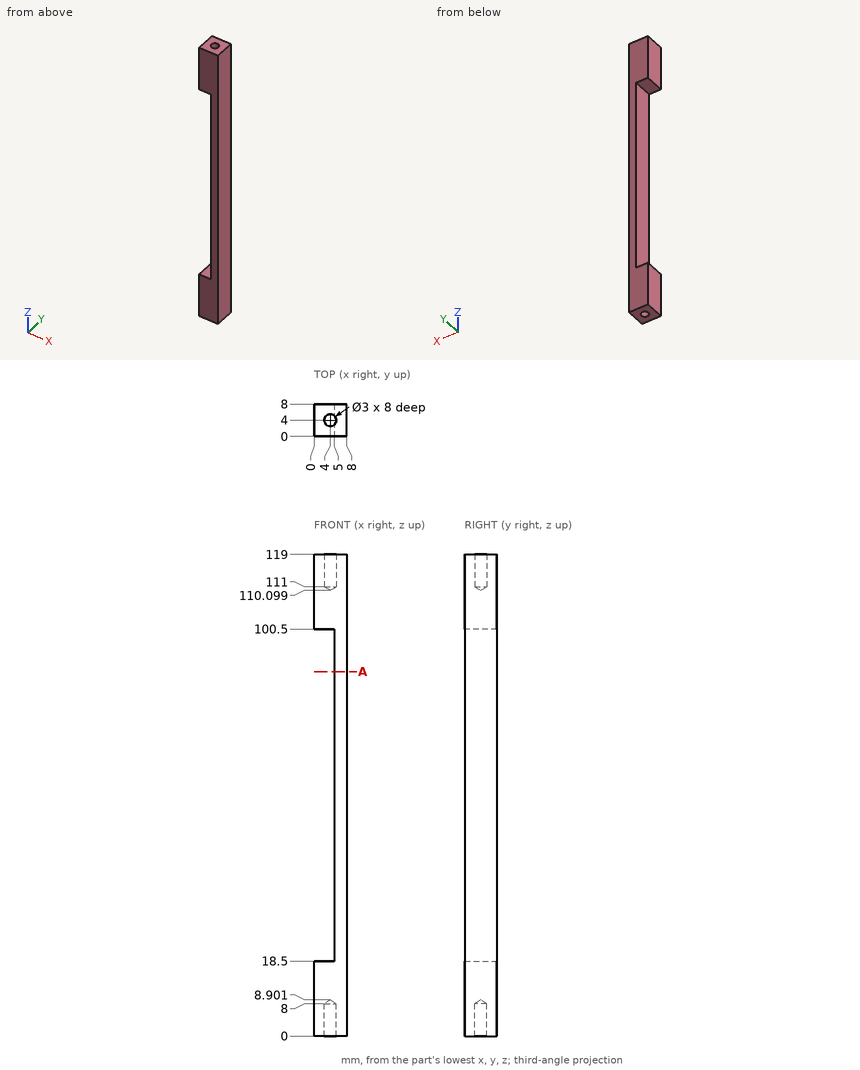
Can you work these out from the drawing? Everything is in mm from the part's minimum corner. Give positions to 0.01 mm unless a question says otherwise; leave off trailing zeros. Loops run counter-clockwise (first coordinate to the right, second up) from the corner with the lowest first, then second, coordinate; pieces in that order, holes last. Notation, with made-up numbers: M 62,54 L 109,54 A12 cw 109,71 Z; hole C 14.5,72.5 d1. An arc over 180 degrees is marked long. Put each result on its own line as item: value. Start each with the question number.
(1) Will this pin go through, and if not, where does the flat tip stop? pin 1 Ø3.5 at (x, y) = (4, 4) entering from -Z.
(2) I want a section at A-A on z = 90. Please give me the cut outline in (x, y).
(3) I need wall thicknesses on line 1 along X through (y, z) = (4, 113.25); line 2 along Z through (x, y) = (3.5, 1). Which ranges of each line are inside material? Lowest first, please. Write a range as [from, to].
Answer block:
1. pin 1: z = 0
2. outline: M 5,0 L 8,0 L 8,8 L 5,8 Z
3. line 1: [0, 2.5], [5.5, 8]
3. line 2: [0, 18.5], [100.5, 119]
